Read the model definition and answer for the solid it produces. Units are mm, in the model's axes. Face numbers are marked on the shaded views. A direction names the side the tool comes from. Give positions to 0.01 mm unless a question says otherwise; leave off trailing zeros. Order: outer loops, then holes, each group sorted by start corner. A loop starts at its lowest first (then second) coordinate and runs counter-clockwise, first axis right, second up. Notation, with made-up numbers: (-15, -12) - (15, -12) arc R23 cw to (15, 25) - close; hole circle Ø7 at (27, 29.5). An arc over 180 degrees is marked (long way). Return JSON: item names as keys, results as strings.
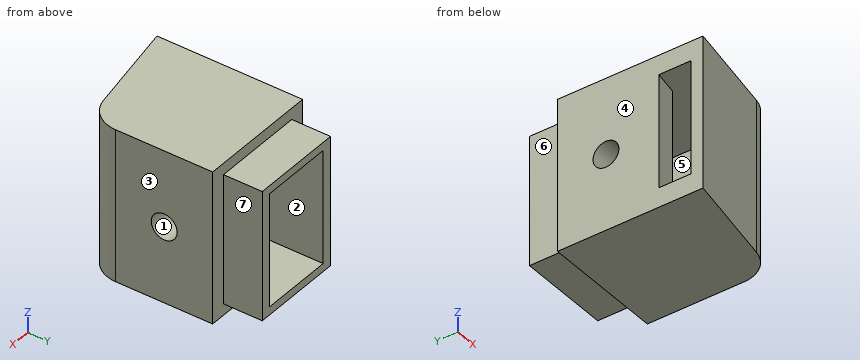
```python
from build123d import *

# Parameters (mm, degrees)
PAD_DEPTH       = 9.41
SKETCH001_W     = 9
SKETCH001_H     = 14
POCKET_DEPTH    = 12
POCKET001_DEPTH = 14
SKETCH003_W     = 11.5
SKETCH003_H     = 16
SKETCH003_W_2   = 9
SKETCH003_H_2   = 14
PAD001_DEPTH    = 4.8
SKETCH004_R     = 1.6
POCKET002_DEPTH = 15.141


with BuildPart() as part:
    # Sketch → Pad (new body, symmetric)
    with BuildSketch(Plane.XY):
        with BuildLine():
            Line((-7.57, 12), (7.57, 12))
            Line((7.57, 12), (7.57, 0))
            ThreePointArc((4.290187, -3.908729), (6.641424, -2.551242), (7.57, 0))
            Line((-7.57, -6), (4.290187, -3.908729))
            Line((-7.57, 0), (-7.57, -6))
            Line((-7.57, 0), (-7.57, 12))
        make_face()
    extrude(amount=PAD_DEPTH, both=True)

    # Sketch001 (on Face1 of Pad) → Pocket (cut)
    with BuildSketch(Plane(origin=(0, 12, 0), x_dir=(-1, 0, 0), z_dir=(0, 1, 0))):
        Rectangle(SKETCH001_W, SKETCH001_H)
    extrude(amount=-POCKET_DEPTH, mode=Mode.SUBTRACT)

    # Sketch002 (on Face7 of Pocket) → Pocket001 (cut)
    with BuildSketch(Plane.XY.offset(-7)):
        with BuildLine():
            Line((-4.5, 0), (-7.57, -0.541324))
            Line((-7.57, -0.541324), (-7.57, -4.5))
            Line((-7.57, -4.5), (2.164299, -2.783581))
            ThreePointArc((2.164299, -2.783581), (3.83872, -1.816853), (4.5, 0))
            Line((-4.5, 0), (4.5, 0))
        make_face()
    extrude(amount=POCKET001_DEPTH, mode=Mode.SUBTRACT)

    # Sketch003 (on Face1 of Pocket001) → Pad001 (join)
    with BuildSketch(Plane(origin=(0, 12, 0), x_dir=(-1, 0, 0), z_dir=(0, 1, 0))):
        Rectangle(SKETCH003_W, SKETCH003_H)
        Rectangle(SKETCH003_W_2, SKETCH003_H_2, mode=Mode.SUBTRACT)
    extrude(amount=PAD001_DEPTH)

    # Sketch004 (on Face2 of Pad001) → Pocket002 (cut, through all)
    with BuildSketch(Plane(origin=(-7.57, 0, 0), x_dir=(0, -1, 0), z_dir=(-1, 0, 0))):
        with Locations((-6, 0)):
            Circle(SKETCH004_R)
    extrude(amount=-POCKET002_DEPTH, mode=Mode.SUBTRACT)


solid = part.part
```
Q1. Consider L1, parallel to Z at x = -3, y = 1.5; L2, parallel to X at y = 10.25, z = 6; L3, parallel to Z at x = -5.25, y = 6. Determine where each line is inside the solid, lowest interval first.
Values:
{"L1": "z = -9.41 to -7, 7 to 9.41", "L2": "x = -7.57 to -4.5, 4.5 to 7.57", "L3": "z = -9.41 to -1.6, 1.6 to 9.41"}
Q2. A cutting plane is placed at C-C (y = 11.25). Write down the section's boundary in (x, z).
Values:
{"outline": "(-7.57, -9.41) - (7.57, -9.41) - (7.57, 9.41) - (-7.57, 9.41) - close; hole (-4.5, -7) - (4.5, -7) - (4.5, 7) - (-4.5, 7) - close"}
Q3. A cutting plane is placed at B-B (z = 0). Write down the section's boundary in (x, y).
Values:
{"outline": "(-7.57, -6) - (4.29, -3.91) arc R3.97 ccw to (7.57, 0) - (7.57, 4.4) - (4.5, 4.4) - (4.5, 0) arc R2.83 cw to (2.16, -2.78) - (-7.57, -4.5) - close; (-7.57, -0.54) - (-4.5, 0) - (-4.5, 4.4) - (-7.57, 4.4) - close; (-7.57, 7.6) - (-4.5, 7.6) - (-4.5, 16.8) - (-5.75, 16.8) - (-5.75, 12) - (-7.57, 12) - close; (4.5, 7.6) - (7.57, 7.6) - (7.57, 12) - (5.75, 12) - (5.75, 16.8) - (4.5, 16.8) - close"}
Q4. For the marked faces 5, 6 and 7, determine the directions among +Z, -Z, +X, -X, +Y, -Y from which every point of the face is accessible in a straight line to the end or side of a thin tool.
Values:
{"face 5": "+Y", "face 6": "+Z, -Z, -X, +Y", "face 7": "+Z, -Z, +X, +Y"}
Q5. A cutting plane is placed at D-D (z = -2.75). Write down the section's boundary in (x, y).
Values:
{"outline": "(-7.57, -6) - (4.29, -3.91) arc R3.97 ccw to (7.57, 0) - (7.57, 12) - (5.75, 12) - (5.75, 16.8) - (4.5, 16.8) - (4.5, 0) arc R2.83 cw to (2.16, -2.78) - (-7.57, -4.5) - close; (-7.57, -0.54) - (-4.5, 0) - (-4.5, 16.8) - (-5.75, 16.8) - (-5.75, 12) - (-7.57, 12) - close"}
Q6. A cutting plane is placed at A-A (y = 6). Write down the section's boundary in (x, z), and give its area (3 significant figures).
Values:
{"outline": "(-7.57, -9.41) - (7.57, -9.41) - (7.57, -1.6) - (4.5, -1.6) - (4.5, -7) - (-4.5, -7) - (-4.5, -1.6) - (-7.57, -1.6) - close; (-7.57, 1.6) - (-4.5, 1.6) - (-4.5, 7) - (4.5, 7) - (4.5, 1.6) - (7.57, 1.6) - (7.57, 9.41) - (-7.57, 9.41) - close", "area": "139 mm²"}
Q7. Determine the mould class of the marked faces 1, 2, 3 and 4 for opening direction X: released by +X, released by -X, zero draft, split by the parting line, or undercut.
Values:
{"face 1": "zero draft", "face 2": "undercut", "face 3": "released by +X", "face 4": "released by -X"}
Q8. Given pin 1 (4 mm diameter, centred on y = 15, z = -1.5, fed in from +X); pin 2 (1.5 mm diameter, centred on x = 1, z = 5, fed in from -Y); pin 3 (2 mm diameter, centred on x = 2.5, z = -6.5, fed in from -Y); pin 4 (1.9 mm diameter, centred on y = 6, z = 0, fed in from +X), each flat-ended and moving along its own axis, determine where each tip first touches the part or whether it passes through.
Values:
{"pin 1": "stops at x = 5.75", "pin 2": "stops at y = -4.62", "pin 3": "stops at y = -4.4", "pin 4": "passes through"}
